Can you work these out from the model? Positions are in its coordinate system, mm. A direction names the side the tool comes from. Round coordinates to 2 decimals unless told otherwise and drop trailing zeros. Order: outer loops, then holes, each group sorted by start corner. A loop starts at its lowest first (then second) coordinate and runs counter-clockwise, first axis right, second up. Notation, with made-up numbers: (42, 39) -> (100, 39) arc R12 ccw to (100, 58) -> close; hole circle Ø9 at (22, 73.5). An arc over 180 degrees is marked (long way). One line per item, written item: value.
```python
from build123d import *

# Parameters (mm, degrees)
SKETCH1_R           = 1.6
BOSS_EXTRUDE1_DEPTH = 3


with BuildPart() as part:
    # Sketch1 → Boss-Extrude1 (new body)
    with BuildSketch(Plane.XY):
        Polygon((0, 15), (72.5, 160), (87.5, 160), (160, 15), (160, 0), (0, 0), align=None)
        with Locations((150, 7.5)):
            Circle(SKETCH1_R, mode=Mode.SUBTRACT)
        with Locations((125, 7.5)):
            Circle(SKETCH1_R, mode=Mode.SUBTRACT)
        with Locations((100, 7.5)):
            Circle(SKETCH1_R, mode=Mode.SUBTRACT)
        with Locations(Location((10, 7.5, 0), (0, 0, 180))):
            Circle(SKETCH1_R, mode=Mode.SUBTRACT)
        with Locations(Location((35, 7.5, 0), (0, 0, 180))):
            Circle(SKETCH1_R, mode=Mode.SUBTRACT)
        with Locations(Location((60, 7.5, 0), (0, 0, 180))):
            Circle(SKETCH1_R, mode=Mode.SUBTRACT)
        with Locations((80, 150)):
            Circle(SKETCH1_R, mode=Mode.SUBTRACT)
        with Locations((80, 115)):
            Circle(SKETCH1_R, mode=Mode.SUBTRACT)
        with Locations((80, 80)):
            Circle(SKETCH1_R, mode=Mode.SUBTRACT)
        with Locations((80, 45)):
            Circle(SKETCH1_R, mode=Mode.SUBTRACT)
        Polygon((72.5, 126.458980338), (72.5, 15), (16.770509831, 15), align=None, mode=Mode.SUBTRACT)
        Polygon((87.5, 15), (137.271498835, 15), (87.5, 126.458980338), align=None, mode=Mode.SUBTRACT)
    extrude(amount=BOSS_EXTRUDE1_DEPTH)


solid = part.part
```
Q1. I want a section at D-D on y = 94. List the corners of the cut face in (x, z) for me.
Answers below:
outline: (39.5, 0) -> (56.27, 0) -> (56.27, 3) -> (39.5, 3) -> close; (72.5, 0) -> (87.5, 0) -> (87.5, 3) -> (72.5, 3) -> close; (101.99, 0) -> (120.5, 0) -> (120.5, 3) -> (101.99, 3) -> close
Q2. Please list where these lines run through material, in increasing order: line 1 along X through (y, z) = (69.5, 1.7); line 2 along Y through (x, z) = (60, 1); line 3 along Y through (x, z) = (80, 0.85).
Answers below:
line 1: 27.25 to 44.02, 72.5 to 87.5, 112.93 to 132.75
line 2: 0 to 5.9, 9.1 to 15, 101.46 to 135
line 3: 0 to 43.4, 46.6 to 78.4, 81.6 to 113.4, 116.6 to 148.4, 151.6 to 160
Q3. I want a section at B-B on x = 23.5. List the corners of the cut face in (y, z) for me.
Answers below:
outline: (0, 0) -> (15, 0) -> (15, 3) -> (0, 3) -> close; (28.46, 0) -> (62, 0) -> (62, 3) -> (28.46, 3) -> close
Q4. I want a section at C-C on z = 2.35. Give the number of separate pieces and of enclosed holes in the cut face, plus the area to 3 significant figures.
Answers below:
separate pieces: 1
enclosed holes: 12
area: 9,130 mm^2
Q5. Will this pin go through, and if not, where does the flat tip stop? pin 1 Ø0.9 at (x, z) = (110.5, 2) entering from +Y.
Answers below:
pin 1: y = 114.9
Q6. I want a section at A-A on y = 122. List the corners of the cut face in (x, z) for me, plus the area to 3 significant figures.
Answers below:
outline: (53.5, 0) -> (70.27, 0) -> (70.27, 3) -> (53.5, 3) -> close; (72.5, 0) -> (87.5, 0) -> (87.5, 3) -> (72.5, 3) -> close; (89.49, 0) -> (106.5, 0) -> (106.5, 3) -> (89.49, 3) -> close
area: 146 mm^2
Q7. On a 3-axis mill with a long thin cutter (end or side, diameter ignored), from which of +Z, -Z, +X, -X, +Y, -Y can I reach the whole of each face in a straight line? I mean faces 1 (the face through (81, 63, 3)), 2 (the face through (44.245, 69.949, 1.479)). Say none if no direction works.
Answers below:
face 1: +Z, +X, -X, +Y, -Y
face 2: +Z, -Z
